Input: part model. Units: mm. Frame: model coordinates. Coordinates: 2 decimals unless noted, no trailing zeros. Loops run counter-clockwise (first coordinate to the right, second up) from the corner with the lowest first, then second, coordinate; pieces in that order, holes last. Notation, with made-up numbers: (-10.75, 51.5) - (22.25, 51.5) arc R17 cw to (22.25, 78.5) - close; hole circle Ø10 at (72.5, 66). An arc over 180 degrees is marked (long way). Answer as CSV lines item,"result". Start each with the question number.
```python
from build123d import *

# Parameters (mm, degrees)
SKETCH_1_R      = 8.5
SKETCH_1_R_2    = 3.5
EXTRUDE_1_DEPTH = 6
FILLET_1_R      = 1
FILLET_2_R      = 1


with BuildPart() as part:
    # 草圖1 → 填料-伸長1 (new body)
    with BuildSketch(Plane(origin=(0, 0, 0), x_dir=(1, 0, 0), z_dir=(0, 1, 0))):
        with Locations(Location((0, 0, 0), (0, 0, 270))):
            Circle(SKETCH_1_R)
        with Locations(Location((0, 0, 0), (0, 0, 270))):
            Circle(SKETCH_1_R_2, mode=Mode.SUBTRACT)
    extrude(amount=EXTRUDE_1_DEPTH)

    # 圓角1
    fillet_1_edges = [part.edges().sort_by_distance(p)[0] for p in [
        (0, 6, -8.5),
        (0, 0, -3.5),
        (0, 6, -3.5),
    ]]
    fillet(fillet_1_edges, radius=FILLET_1_R)

    # 圓角2
    fillet_2_edges = [part.edges().sort_by_distance(p)[0] for p in [
        (0, 0, -8.5),
    ]]
    fillet(fillet_2_edges, radius=FILLET_2_R)


solid = part.part
```
Item 1: Section query C-C, the plane y = 4.4. Output: boundary loops of the cut face in (x, z).
Item 2: Section query A-A, the plane x = 0. Output: boundary loops of the cut face in (y, z), and give its area (3 significant figures).
Item 3: Section query B-B, the plane z = 0. Output: boundary loops of the cut face in (x, y).
Item 4: Draft query along X for faces 1 (the cylindrical face through (8.428, 2.972, -1.107)), 2 (the cylindrical face through (-3.417, 2.972, -0.759)), 3 (the flat face through (0, 6, 5)). Return one class per face: pulls with the +X half, pulls with the -X half, needs draft (parallel to the pull), parting line crosses it, or undercut.
Item 5: Material intervals for probe 1 along X at (y, z) = (3.4, 0); probe 2 along Z at (x, y) = (-4, 1.25); probe 3 along Z at (x, y) = (2, 0.3), sorted ascending.
Item 6: Contact query for flat-ended pins moving along their axis: P1, Ø1, axis at y = 3.5, z = 1.5, coming from the -X side; P2, Ø1.5, axis at x = -1.5, y = 4.5, coming from the +Z side; P3, Ø1, axis at x = -1, y = 4.5, coming from the -Z side. Output: stop coordinate, or through.
Response values:
1,outline,"circle Ø17 at (0, 0); hole circle Ø7 at (0, 0)"
2,outline,"(0, -7.5) arc R1 ccw to (1, -8.5) - (5, -8.5) arc R1 ccw to (6, -7.5) - (6, -4.5) arc R1 ccw to (5, -3.5) - (1, -3.5) arc R1 ccw to (0, -4.5) - close; (0, 4.5) arc R1 ccw to (1, 3.5) - (5, 3.5) arc R1 ccw to (6, 4.5) - (6, 7.5) arc R1 ccw to (5, 8.5) - (1, 8.5) arc R1 ccw to (0, 7.5) - close"
2,area,"58.3 mm²"
3,outline,"(-8.5, 1) arc R1 ccw to (-7.5, 0) - (-4.5, 0) arc R1 ccw to (-3.5, 1) - (-3.5, 5) arc R1 ccw to (-4.5, 6) - (-7.5, 6) arc R1 ccw to (-8.5, 5) - close; (3.5, 1) arc R1 ccw to (4.5, 0) - (7.5, 0) arc R1 ccw to (8.5, 1) - (8.5, 5) arc R1 ccw to (7.5, 6) - (4.5, 6) arc R1 ccw to (3.5, 5) - close"
4,face 1,"parting line crosses it"
4,face 2,"undercut"
4,face 3,"needs draft"
5,probe 1,"x = -8.5 to -3.5, 3.5 to 8.5"
5,probe 2,"z = -7.5 to 7.5"
5,probe 3,"z = -7.97 to -3.21, 3.21 to 7.97"
6,P1,"stops at x = -8.44"
6,P2,"stops at z = 8.47"
6,P3,"stops at z = -8.49"
